from build123d import *

# Parameters (mm, degrees)
F0_R     = 39.5
F0_R_2   = 7.25
F1_DEPTH = 12
F4_W     = 25.5
F4_H     = 66.75
F5_DEPTH = 7
F7_DEPTH = 5


with BuildPart() as f1:
    # F0 (on Top) → F1 (new body)
    with BuildSketch(Plane.XY):
        Circle(F0_R)
        Circle(F0_R_2, mode=Mode.SUBTRACT)
    extrude(amount=F1_DEPTH)

    # F4 (on offset) → F5 (cut)
    with BuildSketch(Plane.XY.offset(2.75)):
        with Locations((0, -16.625)):
            Rectangle(F4_W, F4_H)
    extrude(amount=F5_DEPTH, mode=Mode.SUBTRACT)

    # F6 (on face) → F7 (cut)
    with BuildSketch(Plane.XY.offset(12)):
        with BuildLine():
            Line((6, -36.331318), (6, 0))
            ThreePointArc((6, 0), (0, 6), (-6, 0))
            Line((-6, 0), (-6, -36.331318))
            Line((-6, -36.331318), (6, -36.331318))
        make_face()
    extrude(amount=-F7_DEPTH, mode=Mode.SUBTRACT)


solid = f1.part
Verification items for the finished model (mm, model axes). A direction names the side the tool comes from. Coordinates: 2 decimals unless noted, no trailing zeros. Loops run counter-clockwise (first coordinate to the right, second up) from the corner with the lowest first, then second, coordinate; pieces in that order, holes last. Notation, with made-up numbers: (21.25, 68.5) -> (78.25, 68.5) arc R25 ccw to (78.25, 95.5) -> close; hole circle Ø2 at (-8.5, 14). An arc over 180 degrees is marked (long way). Answer as CSV lines item,"result".
1) Thickness scan on L1, parallel to Y at x = 0, z = 1.25; L2, parallel to Y at x = 0, z = 10.9; L3, parallel to X at y = -14.5, z = 10.75. Record the ranges inside material, lowest first. Write a range as from..to.
Found:
L1,"y = -39.5..-7.25, 7.25..39.5"
L2,"y = -39.5..-36.33, 7.25..39.5"
L3,"x = -36.74..-6, 6..36.74"
2) Tool access check on faces 1 (the flat face through (12.75, -11, 6)), 2 (the flat face through (-6, -20, 11)), 3 (the flat face through (-1, -8, 0)). Record the directions out of +Z, -Z, +X, -X, +Y, -Y that give a thin tool (end or side, any length) a straight path to the whole face; none if there is none.
Found:
face 1,"-Y"
face 2,"+Z"
face 3,"-Z, +X, -X, +Y, -Y"
3) Cross-section at A-A, the plane x = 0. Record the cut outline in (y, z), then the cut area to 3 significant figures.
Found:
outline,"(-39.5, 0) -> (-7.25, 0) -> (-7.25, 2.75) -> (-39.5, 2.75) -> close; (-39.5, 9.75) -> (-36.33, 9.75) -> (-36.33, 12) -> (-39.5, 12) -> close; (7.25, 0) -> (39.5, 0) -> (39.5, 12) -> (7.25, 12) -> (7.25, 9.75) -> (16.75, 9.75) -> (16.75, 2.75) -> (7.25, 2.75) -> close"
area,"416 mm2"
4) Release check for a two-part mould opening along Z. For faces 4 (the flat face through (6, -20, 11)), 5 (the flat face through (8, 1, 12)), 6 (the flat face through (-9, -5, 9.75)) record: +Z half, -Z half, draft (parallel to the pull), parting line (faces both ways), or undercut.
Found:
face 4,"draft"
face 5,"+Z half"
face 6,"undercut"
5) Cross-section at B-B, the plane y = 0. Record the cut outline in (x, z), then the cut area to 3 significant figures.
Found:
outline,"(-39.5, 0) -> (-7.25, 0) -> (-7.25, 2.75) -> (-12.75, 2.75) -> (-12.75, 9.75) -> (-7.25, 9.75) -> (-7.25, 12) -> (-39.5, 12) -> close; (7.25, 0) -> (39.5, 0) -> (39.5, 12) -> (7.25, 12) -> (7.25, 9.75) -> (12.75, 9.75) -> (12.75, 2.75) -> (7.25, 2.75) -> close"
area,"697 mm2"
6) Depth check by flat-ended pin: pin 1 (5.5 mm diameter, centred on x = 2, z = 5, fed in from -Y); pin 2 (5.5 mm diameter, centred on y = -13.5, z = 7, fed in from +X); pin 3 (3 mm diameter, centred on y = -2, z = 10.5, fed in from -X). Enter the tip coordinate at first touch or a pass-through.
Found:
pin 1,"stops at y = -39.5"
pin 2,"stops at x = 38.01"
pin 3,"stops at x = -39.5"
7) Cross-section at C-C, the plane z = 1.75. Record the cut outline in (x, y), then the cut area to 3 significant figures.
Found:
outline,"circle Ø79 at (0, 0); hole circle Ø14.5 at (0, 0)"
area,"4,740 mm2"
8) Cross-section at D-D, the plane x = 9. Record the cut outline in (y, z), then the cut area to 3 significant figures.
Found:
outline,"(-38.46, 0) -> (38.46, 0) -> (38.46, 12) -> (-38.46, 12) -> (-38.46, 9.75) -> (16.75, 9.75) -> (16.75, 2.75) -> (-38.46, 2.75) -> close"
area,"537 mm2"
